```python
from build123d import *

# Parameters (mm, degrees)
SKETCH1_W      = 146.737083443
SKETCH1_H      = 152.4
SKETCH1_R      = 2.814870932
EXTRUDE1_DEPTH = 12.7
SKETCH2_R      = 3.175
SKETCH2_R_2    = 3.301739158
EXTRUDE2_DEPTH = 192.148134104
SKETCH3_R      = 9.711530505
EXTRUDE3_DEPTH = 7.62
FILLET1_R      = 2.54


with BuildPart() as part:
    # Sketch1 → Extrude1 (new body)
    with BuildSketch(Plane.XY):
        with Locations((39.132231405, -76.2)):
            Rectangle(SKETCH1_W, SKETCH1_H)
        with Locations((-22.131450225, -19.446874936)):
            Circle(SKETCH1_R, mode=Mode.SUBTRACT)
    extrude(amount=EXTRUDE1_DEPTH)

    # Sketch2 → Extrude2 (cut, through all)
    with BuildSketch(Plane(origin=(-5.4e-08, -8.6e-08, -12.901274016), x_dir=(-1.0, 0, 4.210511821155492e-09), z_dir=(-4.210511821155492e-09, -6.669209052807934e-09, -1.0))):
        with Locations(Location((-100.395913074, -19.446875, 0), (0, 0, 90))):
            Circle(SKETCH2_R)
        with Locations(Location((-100.395913114, -56.753124936, 0), (0, 0, 90))):
            Circle(SKETCH2_R_2)
        with Locations(Location((-100.395913114, -94.091124936, 0), (0, 0, 90))):
            Circle(SKETCH2_R)
        with Locations(Location((-100.395913114, -131.429124936, 0), (0, 0, 90))):
            Circle(SKETCH2_R)
        with Locations(Location((22.131450318, -56.753125108, 0), (0, 0, 90))):
            Circle(SKETCH2_R)
        with Locations(Location((22.131450318, -94.091124936, 0), (0, 0, 90))):
            Circle(SKETCH2_R)
        with Locations(Location((22.131450318, -131.429124936, 0), (0, 0, 90))):
            Circle(SKETCH2_R)
        with Locations(Location((22.131450278, -19.446875021, 0), (0, 0, 90))):
            Circle(SKETCH2_R)
    extrude(amount=-EXTRUDE2_DEPTH, mode=Mode.SUBTRACT)

    # Sketch3 → Extrude3 (add)
    # profile 1 of 2: a face of its own
    with BuildSketch(Plane.XY.offset(12.7)):
        with BuildLine():
            Line((112.500773126, -152.4), (-34.236310317, -152.4))
            Line((-34.236310317, -152.4), (6.055614242, -212.627943895))
            ThreePointArc((6.055614242, -212.627943895), (39.132231405, -230.295835259), (72.208848567, -212.627943895))
            Line((72.208848567, -212.627943895), (112.500773126, -152.4))
        make_face()
        with Locations((39.132231405, -190.5)):
            Circle(SKETCH3_R, mode=Mode.SUBTRACT)
    # profile 2 of 2: a face of its own
    with BuildSketch(Plane.XY.offset(12.7)):
        with BuildLine():
            Line((112.500773126, 0), (-34.236310317, 0))
            Line((-34.236310317, 0), (6.055614242, 60.227943895))
            ThreePointArc((6.055614242, 60.227943895), (39.132231405, 77.895835259), (72.208848567, 60.227943895))
            Line((72.208848567, 60.227943895), (112.500773126, 0))
        make_face()
        with Locations((39.132231405, 38.1)):
            Circle(SKETCH3_R, mode=Mode.SUBTRACT)
    extrude(amount=-EXTRUDE3_DEPTH)

    # Fillet1
    fillet1_edges = [part.edges().sort_by_distance(p)[0] for p in [
        (39.132231405, -152.4, 5.08),
        (39.132231405, 0, 5.08),
    ]]
    fillet(fillet1_edges, radius=FILLET1_R)


solid = part.part
```
Input: part model. Units: mm. Frame: model coordinates. A direction names the side the tool comes from. Coordinates: 2 decimals unless noted, no trailing zeros. Write each loop counter-clockwise with the first axis right and the second up, starting at its lowest first coordinate (ties: lowest second). Pieces come first, ordered by that corner, then holes. Notation, with made-up numbers: (21.5, -3) -> (41.5, -3) arc R35 cw to (41.5, 31) -> close; hole circle Ø4 at (27, 24.5). An arc over 180 degrees is marked (long way). Write each question's results on one line, items separated by ' | '.
Item 1: Mould query, pull axis Y, two halves, no side actions, for faces 3 (the cylindrical face through (-23.347, -128.496, 6.261)), 4 (the flat face through (-14.372, 29.692, 8.82)), 5 (the cylindrical face through (38.586, -230.292, 8.943)). Classes: +Y half, -Y half, draft (parallel to the pull), parting line (faces both ways), or undercut.
Conclusion:
face 3: undercut | face 4: +Y half | face 5: -Y half
Item 2: Section query C-C on z = 8. Count the separate pieces of the cut face and the enclosed holes in it, plus the area to 3 significant figures.
Conclusion:
separate pieces: 1 | enclosed holes: 10 | area: 36,000 mm^2
Item 3: Set-up query: faces 1 (the flat face through (38, -175, 5.08)), 2 (the flat face through (92.07, 30.54, 8.82)). Return all of +Z, -Z, +X, -X, +Y, -Y with unobstructed straight access to the full face (end or side cutting, diameter ignored); none if empty.
Conclusion:
face 1: -Z, +X, -X, -Y | face 2: +Z, -Z, +X, +Y
Item 4: Pin query (flat end, axial travel): pin 1 Ø6 at (x, y) = (100.4, -56.75) entering from +Z; pin 2 Ø8.5 at (x, y) = (100.4, -19.45) entering from -Z; pin 3 Ø4 at (x, z) = (68.5, 5) entering from +Y; pin 4 Ø22.5 at (x, y) = (15, -209) entering from -Z. Return the tip coordinate at first contact, or that it passes through.
Conclusion:
pin 1: passes through | pin 2: stops at z = 0 | pin 3: stops at y = 66.99 | pin 4: stops at z = 5.08
Item 5: Section query D-D on x = 11.5. Return loops of the section in (y, z), plus the area to 3 significant figures.
Conclusion:
outline: (-219.14, 5.08) -> (-154.94, 5.08) arc R2.54 cw to (-152.4, 2.54) -> (-152.4, 0) -> (0, 0) -> (0, 2.54) arc R2.54 cw to (2.54, 5.08) -> (66.74, 5.08) -> (66.74, 12.7) -> (-219.14, 12.7) -> close | area: 2,960 mm^2
Item 6: Material intervals for probe 1 along X at (y, z) = (-132, 6.25); probe 2 along Y at (x, z) = (102, 5.5); probe 3 along Z at (x, y) = (14, -166), sorted ascending.
Conclusion:
probe 1: x = -34.24 to -25.25, -19.01 to 97.27, 103.52 to 112.5 | probe 2: y = -168.1 to -134.17, -128.69 to -96.83, -91.35 to -59.64, -53.87 to -22.19, -16.71 to 15.7 | probe 3: z = 5.08 to 12.7
Item 7: Section query B-B on y = 38.1. Return loops of the section in (x, z), plus the area to 3 significant figures.
Conclusion:
outline: (-8.75, 5.08) -> (29.42, 5.08) -> (29.42, 12.7) -> (-8.75, 12.7) -> close; (48.84, 5.08) -> (87.01, 5.08) -> (87.01, 12.7) -> (48.84, 12.7) -> close | area: 582 mm^2
Item 8: Section query A-A on x = 45. Return loops of the section in (y, z), plus the area to 3 significant figures.
Conclusion:
outline: (-229.86, 5.08) -> (-198.24, 5.08) -> (-198.24, 12.7) -> (-229.86, 12.7) -> close; (-182.76, 5.08) -> (-154.94, 5.08) arc R2.54 cw to (-152.4, 2.54) -> (-152.4, 0) -> (0, 0) -> (0, 2.54) arc R2.54 cw to (2.54, 5.08) -> (30.36, 5.08) -> (30.36, 12.7) -> (-182.76, 12.7) -> close; (45.84, 5.08) -> (77.46, 5.08) -> (77.46, 12.7) -> (45.84, 12.7) -> close | area: 2,880 mm^2
